Part model, mm, in its own coordinate system. A direction names the side the tool comes from. Round coordinates to 2 decimals unless told otherwise and drop trailing zeros. Loops run counter-clockwise (first coordinate to the right, second up) from the corner with the lowest first, then second, coordinate; pieces in that order, holes last. Notation, with made-up numbers: (72.5, 14) - (124.5, 14) arc R10 cw to (124.5, 33) - close; hole circle Ø3 at (-5, 75.25). An arc over 180 degrees is marked (long way). Put each result on its own line as item: value.
from build123d import *

# Parameters (mm, degrees)
SKETCH_1_W          = 29
SKETCH_1_H          = 39
EXTRUDE_1_DEPTH     = 16
SKETCH_2_R          = 12.25
CUT_EXTRUDE_1_DEPTH = 14
SKETCH_3_R          = 6.75
CUT_EXTRUDE_2_DEPTH = 14
SKETCH_4_R          = 1.5
CUT_EXTRUDE_3_DEPTH = 14
SKETCH_5_R          = 1.5
CUT_EXTRUDE_4_DEPTH = 10
CUT_EXTRUDE_START   = -10
SKETCH_6_R          = 1.5
CUT_EXTRUDE_6_DEPTH = 10


with BuildPart() as part:
    # 草图1 → 凸台-拉伸1 (new body)
    with BuildSketch(Plane.XY):
        with Locations((13.362025316, 5)):
            Rectangle(SKETCH_1_W, SKETCH_1_H)
    extrude(amount=EXTRUDE_1_DEPTH)

    # 草图2 → 切除-拉伸1 (cut)
    with BuildSketch(Plane.XY.offset(16)):
        with Locations((13.362025316, 5)):
            Circle(SKETCH_2_R)
    extrude(amount=-CUT_EXTRUDE_1_DEPTH, mode=Mode.SUBTRACT)

    # 草图3 → 切除-拉伸2 (cut)
    with BuildSketch(Plane(origin=(0, 0, 0), x_dir=(-1, 0, 0), z_dir=(0, 0, -1))):
        with Locations((-13.362025316, 5)):
            Circle(SKETCH_3_R)
    extrude(amount=-CUT_EXTRUDE_2_DEPTH, mode=Mode.SUBTRACT)

    # 草图4 → 切除-拉伸3 (cut)
    with BuildSketch(Plane(origin=(0, 0, 0), x_dir=(-1, 0, 0), z_dir=(0, 0, -1))):
        with Locations((-13.362025316, 14.5)):
            Circle(SKETCH_4_R)
        with Locations((-5.134783981, 9.75)):
            Circle(SKETCH_4_R)
        with Locations((-5.134783981, 0.25)):
            Circle(SKETCH_4_R)
        with Locations((-13.362025316, -4.5)):
            Circle(SKETCH_4_R)
        with Locations((-21.589266652, 0.25)):
            Circle(SKETCH_4_R)
        with Locations((-21.589266652, 9.75)):
            Circle(SKETCH_4_R)
    extrude(amount=-CUT_EXTRUDE_3_DEPTH, mode=Mode.SUBTRACT)

    # 草图5 → 切除-拉伸4 (cut)
    with BuildSketch(Plane.ZY.offset(1.137974684)):
        with Locations((12.5, 21)):
            Circle(SKETCH_5_R)
        with Locations(Location((3.5, 21, 0), (0, 0, 180))):
            Circle(SKETCH_5_R)
        with Locations(Location((12.5, -11, 0), (0, 0, 180))):
            Circle(SKETCH_5_R)
        with Locations((3.5, -11)):
            Circle(SKETCH_5_R)
    extrude(amount=-CUT_EXTRUDE_4_DEPTH, mode=Mode.SUBTRACT)

    # 草图6 → 切除-拉伸6 (cut)
    with BuildSketch(Plane(origin=(27.862025316, 0, 0), x_dir=(0, 0, -1), z_dir=(1, 0, 0)).offset(CUT_EXTRUDE_START)):
        with Locations((-12.5, -11)):
            Circle(SKETCH_6_R)
        with Locations(Location((-3.5, -11, 0), (0, 0, 180))):
            Circle(SKETCH_6_R)
        with Locations((-3.5, 21)):
            Circle(SKETCH_6_R)
        with Locations(Location((-12.5, 21, 0), (0, 0, 180))):
            Circle(SKETCH_6_R)
    extrude(amount=CUT_EXTRUDE_6_DEPTH, mode=Mode.SUBTRACT)


solid = part.part
1. Band-saw the part on D-D (x = 22.5). List the corners of the cut face in (y, z), plus the area to 3 significant figures.
A:
outline: (-14.5, 0) - (-0.94, 0) - (-0.94, 2) - (-3.16, 2) - (-3.16, 16) - (-14.5, 16) - close; (1.44, 0) - (8.56, 0) - (8.56, 2) - (1.44, 2) - close; (10.94, 0) - (24.5, 0) - (24.5, 16) - (13.16, 16) - (13.16, 2) - (10.94, 2) - close; hole circle Ø3 at (-11, 3.5); hole circle Ø3 at (-11, 12.5); hole circle Ø3 at (21, 3.5); hole circle Ø3 at (21, 12.5)
area: 358 mm²
2. Probe line 1 along Y through (x, z) = (5.5, 3.5); line 2 along Y through (x, z) = (18.75, 15); line 3 along Z through (x, y) = (1.5, 22). List the from-to ranges inside material, lowest first. Write a range as [from, to].
A:
line 1: y = [-14.5, -12.5], [-9.5, -4.39], [14.39, 19.5], [22.5, 24.5]
line 2: y = [-14.5, -6], [16, 24.5]
line 3: z = [0, 2.38], [4.62, 11.38], [13.62, 16]
3. Band-saw the part on B-B (z = 3.5). List the corners of the cut face in (x, y).
A:
outline: (-1.14, -14.5) - (27.86, -14.5) - (27.86, -12.5) - (17.86, -12.5) - (17.86, -9.5) - (27.86, -9.5) - (27.86, 19.5) - (17.86, 19.5) - (17.86, 22.5) - (27.86, 22.5) - (27.86, 24.5) - (-1.14, 24.5) - (-1.14, 22.5) - (8.86, 22.5) - (8.86, 19.5) - (-1.14, 19.5) - (-1.14, -9.5) - (8.86, -9.5) - (8.86, -12.5) - (-1.14, -12.5) - close; hole circle Ø24.5 at (13.36, 5)
4. Two-plate mould, pull along Y, no slides. Class faces 4 (the flat face through (13, -14.5, 8)), 5 (the flat face through (7, 10, 0)), 6 (the cylindrical face through (14.86, 14.57, 0.99)): pulls with the +Y half, pulls with the -Y half, needs draft (parallel to the pull), parting line crosses it, or undercut.
A:
face 4: pulls with the -Y half
face 5: needs draft
face 6: undercut
5. Band-saw the part on A-A (y = 5). List the corners of the cut face in (x, z), plus the area to 3 significant figures.
A:
outline: (-1.14, 0) - (6.61, 0) - (6.61, 2) - (1.11, 2) - (1.11, 16) - (-1.14, 16) - close; (20.11, 0) - (27.86, 0) - (27.86, 16) - (25.61, 16) - (25.61, 2) - (20.11, 2) - close
area: 94.0 mm²
6. Pin check, flat tips, straight feed: P1, Ø1.8, axis at x = 13.36, y = -4.5, coming from the -Z side; P2, Ø2.5, axis at y = 21, z = 3.5, coming from the -X side. Stop position of each tip, or through.
A:
P1: passes through
P2: stops at x = 8.86
7. Band-saw the part on C-C (x = 9.5). List the corners of the cut face in (y, z), plus the area to 3 significant figures.
A:
outline: (-14.5, 0) - (-0.54, 0) - (-0.54, 2) - (-6.63, 2) - (-6.63, 16) - (-14.5, 16) - close; (10.54, 0) - (24.5, 0) - (24.5, 16) - (16.63, 16) - (16.63, 2) - (10.54, 2) - close
area: 276 mm²
8. Tool access for faces 1 (the flat face through (19, 0, 2)), 2 (the cylindrical face through (22.792, 19.513, 12.305)), 3 (the flat face through (8.862, 21, 12)): list every direction of +Z, -Z, +X, -X, +Y, -Y with a clear straight run to the whole face (end or side of a thin tool).
A:
face 1: +Z
face 2: +X
face 3: -X
